Input: part model. Units: mm. Frame: model coordinates. A direction names the side the tool comes from. Coordinates: 2 decimals unless noted, no trailing zeros. Loops run counter-clockwise (first coordinate to the right, second up) from the corner with the lowest first, then second, coordinate; pieces in that order, holes last. Notation, with made-up numbers: (41, 10.25) -> (100, 10.25) arc R22 ccw to (100, 36.25) -> close; hole circle Ø4 at (28, -1). An arc over 180 degrees is marked (long way). Put each result on its own line as item: value. Start each with the question number.
1) Cut plane A-A (y = 6.5). Return the cut outline in (x, z) (1 decimal).
2) Contact query for flat-ended pins moving along their axis: P1, Ø1.5, axis at x = 16, y = 1, coming from the -Z side; P2, Ø2, axis at x = 4.5, z = -2.5, coming from the +Y side; P3, Ø3, axis at y = 4, z = 2, coming from the -X side (3 decimals). Output: stop coordinate, or through.
3) Pull-direction query (Y, two-part tool) for faces 4 (the flat face through (22.225, 10, 0)), 5 (the flat face through (0, -1.27, 3)), 6 (the flat face through (-17, 11.43, 0)), 7 (the flat face through (-18, 0, 0)); classes: pulls with the +Y half, pulls with the -Y half, needs draft (parallel to the pull), parting line crosses it, or undercut.
4) Cut plane B-B (z = -0.75). State how many separate pieces and enclosed holes the cut face has, plus the area to 3 significant figures.
5) Cut plane D-D (x = 0). Return the cut outline in (y, z).
6) Set-up query: faces 1 (the flat face through (20.955, 1, 0)), 2 (the flat face through (3, 1.27, 0)), 3 (the flat face through (22, 1.905, 0)). Return all of +Z, -Z, +X, -X, +Y, -Y with unobstructed straight access to the full face (end or side cutting, diameter ignored); none if empty.
7) Material intervals for L1, parallel to X at y = 10, z = 0 (3 decimals); L2, parallel to X at y = 10.75, z = 1.5 (3 decimals); L3, parallel to X at y = 3.5, z = -3 (3 decimals), sorted ascending.
from build123d import *

# Parameters (mm, degrees)
F0_R     = 0.396875
F0_W     = 25.4
F0_H     = 2.54
F1_DEPTH = 4.7625
F2_R     = 2.38125
F3_DEPTH = 5.969


# Not quite as in the source:
# - a length typed as a fraction of an inch, garbled in the dataset ("3 / 203.2 mm" for 3/8 in), is restored
# - a feature names something its author has since deleted; it is built from what else it names


with BuildPart() as f1:
    # F0 (on Top) → F1 (new body, symmetric)
    with BuildSketch(Plane.XY):
        Polygon((-12.7, 11.43), (-22.225, 11.43), (-22.225, 8.255), (-20.955, 8.255), (-20.955, 10.16), (-14.605, 10.16), (-14.605, 0), (-20.955, 0), (-20.955, 1.905), (-22.225, 1.905), (-22.225, -1.27), (-12.7, -1.27), (-12.7, 1.27), align=None)
        with Locations((-21.59, 1.397)):
            Circle(F0_R, mode=Mode.SUBTRACT)
        with Locations((-21.59, 8.763)):
            Circle(F0_R, mode=Mode.SUBTRACT)
        Rectangle(F0_W, F0_H)
        Polygon((12.7, 11.43), (12.7, 1.27), (12.7, -1.27), (22.225, -1.27), (22.225, 1.905), (20.955, 1.905), (20.955, 0), (14.605, 0), (14.605, 10.16), (20.955, 10.16), (20.955, 8.255), (22.225, 8.255), (22.225, 11.43), align=None)
        with Locations((21.59, 1.397)):
            Circle(F0_R, mode=Mode.SUBTRACT)
        with Locations((21.59, 8.763)):
            Circle(F0_R, mode=Mode.SUBTRACT)
    extrude(amount=F1_DEPTH, both=True)

    # F2 (on face) → F3 (cut)
    with BuildSketch(Plane(origin=(0, 1.27, 0), x_dir=(-1, 0, 0), z_dir=(0, 1, 0))):
        Circle(F2_R)
    extrude(amount=-F3_DEPTH, mode=Mode.SUBTRACT)


solid = f1.part
Results found:
1. outline: (-14.6, -4.8) -> (-12.7, -4.8) -> (-12.7, 4.8) -> (-14.6, 4.8) -> close; (12.7, -4.8) -> (14.6, -4.8) -> (14.6, 4.8) -> (12.7, 4.8) -> close
2. P1: passes through
2. P2: stops at y = 1.27
2. P3: stops at x = -14.605
3. face 4: needs draft
3. face 5: pulls with the -Y half
3. face 6: pulls with the +Y half
3. face 7: undercut
4. separate pieces: 2
4. enclosed holes: 4
4. area: 148 mm2
5. outline: (-1.27, -4.76) -> (1.27, -4.76) -> (1.27, -2.38) -> (-1.27, -2.38) -> close; (-1.27, 2.38) -> (1.27, 2.38) -> (1.27, 4.76) -> (-1.27, 4.76) -> close
6. face 1: +Z, -Z
6. face 2: +Z, -Z, +Y
6. face 3: +Z, -Z, +X
7. L1: x = -22.225 to -20.955, -14.605 to -12.7, 12.7 to 14.605, 20.955 to 22.225
7. L2: x = -22.225 to -12.7, 12.7 to 22.225
7. L3: x = -14.605 to -12.7, 12.7 to 14.605
